Design review of the part shown in the three views and the two pictorial views. Dimensions are in mm from the part's minimum x, y and z. A direction names the side the tool comes from. Round coordinates to 2 decimals unless told otherwise and drop trailing zeros. Loops run counter-clockwise (first coordinate to the right, second up) from the corner with the lowest first, then second, coordinate; pieces in that order, holes last.
1. Consider section D-D on z = 90. State the section outline as (x, y) points (1 decimal), then the cut area to 3 significant figures.
2. Tool access review of the marked faces 4, 5 and 6: name each direction out of +Z, -Z, +X, -X, +Y, -Y from which nothing blocks a thin tool from reaching the whole face with its end or side.
3. Consider section C-C on x = 50. State the section outline as (y, z) points.
4. Consider section A-A on z = 50. State the section outline as (x, y) points.
5. Clearance check with flat-ended pins moving along their axes: pin 1 Ø8 at (y, z) = (45, 55.5) entering from +X; pin 2 Ø3 at (x, y) = (35.5, 37) entering from -Z; pin 3 Ø3 at (y, z) = (35, 76) entering from +X; pin 4 Ø21 at (y, z) = (90, 50) entering from -X. State where each tip first meets the part, or that it passes through.
6. Draft analysis for pull direction X (two halves, no side actions). For the marked faces 1, 2 and 3, state which applies: released by +X, released by -X, zero draft, split by the parting line, or undercut.
7. To check wall thickness, follow line 1 along Y through (x, z) = (92.25, 50); line 2 along Y through (x, z) = (87, 40.5); line 3 along X through (y, z) = (74, 80). State the ranges of each line that lie inside material, in increasing order.
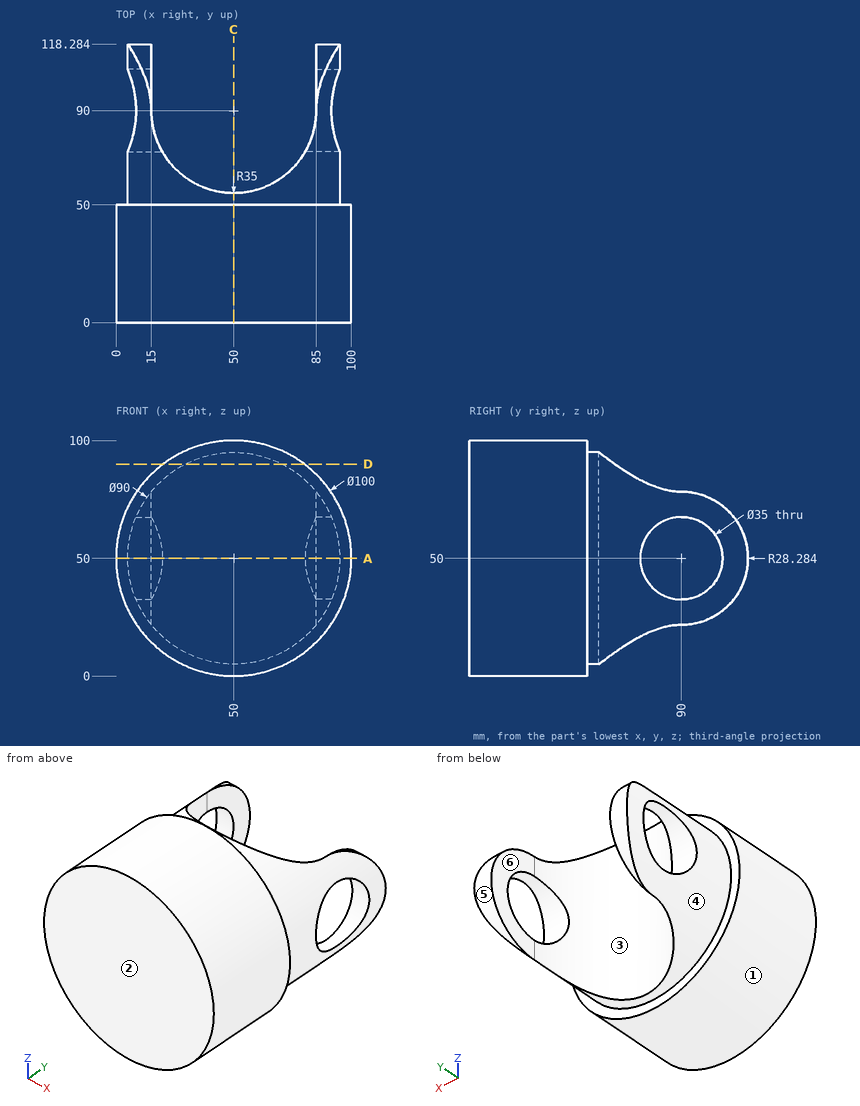
Resolved:
1. outline: (20, 0) - (80, 0) - (80, 50) - (70.6, 50) - (70.6, 61.7) arc R35 cw to (29.4, 61.7) - (29.4, 50) - (20, 50) - close
1. area: 3,290 mm2
2. face 4: +Y
2. face 5: +X, -X, +Y
2. face 6: +Z, -Z, +Y
3. outline: (0, 0) - (50, 0) - (50, 5) - (55, 5) - (55, 95) - (50, 95) - (50, 100) - (0, 100) - close
4. outline: (0, 0) - (100, 0) - (100, 50) - (95, 50) - (95, 72.5) - (80.31, 72.5) arc R35 cw to (19.69, 72.5) - (5, 72.5) - (5, 50) - (0, 50) - close; (5, 107.5) - (15, 107.5) - (15, 118.28) - (5, 118.28) - close; (85, 107.5) - (95, 107.5) - (95, 118.28) - (85, 118.28) - close
5. pin 1: stops at x = 99.98
5. pin 2: stops at z = 1.72
5. pin 3: stops at x = 93.59
5. pin 4: passes through
6. face 1: split by the parting line
6. face 2: zero draft
6. face 3: undercut
7. line 1: y = 0 to 72.5, 107.5 to 118.28
7. line 2: y = 0 to 75.3, 104.7 to 116.64
7. line 3: x = 16.46 to 18.87, 81.13 to 83.54
